Input: part model. Units: mm. Frame: model coordinates. A direction names the side the tool comes from. Coordinates: 2 decimals unless noted, no trailing zeros. Put each result on its own line as item: value. Start each with the question number.
1) Contact query for flat-ended pins moving along their axis: P1, Ø2, axis at x = -1.5, y = -1, coming from the -Z side; P2, Ø3, axis at x = 4, y = -3, coming from the +Z side; P3, Ø2, axis at y = 1.5, z = 10, coming from the +X side; P4, Ø1, axis at y = -7, z = 12, coming from the -X side. Output: stop coordinate, or through.
2) Material intervals for L1, parallel to Y at x = -3, z = 9.5; L2, parallel to Y at x = 3.25, z = 1.5; L3, parallel to X at y = -2.25, z = 4.25, sorted ascending.
3) Set-up query: faces 4 (the flat face through (-4, 0, 5)), 5 (the cylindrical face through (-1.859, -9.919, 24.032)), 6 (the cylindrical face through (3.098, -6.416, 20.157)), 7 (the cylindrical face through (-1.941, -3.786, 27.573)), 8 (the cylindrical face through (4.241, -6.849, 25.805)). Return all of +Z, -Z, +X, -X, +Y, -Y with unobstructed straight access to the full face (end or side cutting, diameter ignored); none if empty.
4) Pull-direction query (X, two-part tool) for faces 1 (the cylindrical face through (3.1, 2.44, 5.34)), 2 (the flat face through (-5.05, -6.98, 25.99)), 3 (the cylindrical face through (5.359, -6.849, 25.805)); classes: pulls with the +X half, pulls with the -X half, needs draft (parallel to the pull), parting line crosses it, or undercut.
from build123d import *

# Parameters (mm, degrees)
CUT_EXTRUDE1_DEPTH = 10
CUT_EXTRUDE2_DEPTH = 10
FILLET1_R          = 0.8


with BuildPart() as part:
    # Sweep1: sweep along a path in Sketch2
    with BuildLine(Plane(origin=(0, 0, 0), x_dir=(0, 0, -1), z_dir=(1, 0, 0))) as sweep1_path:
        Line((0, 0), (-10, 0))
        ThreePointArc((-10, 0), (-13.799332082, -0.500191558), (-17.339745962, -1.966679003))
        Line((-17.339745962, -1.966679003), (-26, -6.966679003))
    # Sketch1 → Sweep1 (sweep)
    with BuildSketch(Plane.XY):
        with BuildLine():
            Line((-5.6, 4.9), (1, 4.9))
            ThreePointArc((1, 4.9), (4.252691193, 3.552691193), (5.6, 0.3))
            Line((5.6, 0.3), (5.6, -0.3))
            ThreePointArc((5.6, -0.3), (4.252691193, -3.552691193), (1, -4.9))
            Line((1, -4.9), (-5.6, -4.9))
            Line((-5.6, -4.9), (-5.6, 4.9))
        make_face()
        Polygon((2.655811238, 0), (1.327905619, 2.3), (-1.327905619, 2.3), (-2.655811238, 0), (-1.327905619, -2.3), (1.327905619, -2.3), align=None, mode=Mode.SUBTRACT)
    sweep(path=sweep1_path.line)

    # Sketch3 → Cut-Extrude1 (cut)
    with BuildSketch(Plane(origin=(0, 0, 0), x_dir=(-1, 0, 0), z_dir=(0, 0, -1))):
        with BuildLine():
            Line((4, -3.3), (4, 3.3))
            Line((4, 3.3), (-1, 3.3))
            ThreePointArc((-1, 3.3), (-3.121320344, 2.421320344), (-4, 0.3))
            Line((-4, 0.3), (-4, -0.3))
            ThreePointArc((-4, -0.3), (-3.121320344, -2.421320344), (-1, -3.3))
            Line((-1, -3.3), (4, -3.3))
        make_face()
    extrude(amount=-CUT_EXTRUDE1_DEPTH, mode=Mode.SUBTRACT)

    # Sketch4 → Cut-Extrude2 (cut)
    with BuildSketch(Plane(origin=(0, -13, 22.516660498), x_dir=(1, 0, 0), z_dir=(0, -0.5000000000000009, 0.8660254037844382))):
        with BuildLine():
            Line((-4, 10.266679003), (-4, 3.666679003))
            Line((-4, 3.666679003), (1, 3.666679003))
            ThreePointArc((1, 3.666679003), (3.121320344, 4.54535866), (4, 6.666679003))
            Line((4, 6.666679003), (4, 7.266679003))
            ThreePointArc((4, 7.266679003), (3.121320344, 9.387999347), (1, 10.266679003))
            Line((1, 10.266679003), (-4, 10.266679003))
        make_face()
    extrude(amount=-CUT_EXTRUDE2_DEPTH, mode=Mode.SUBTRACT)

    # Fillet1
    fillet1_edges = [part.edges().sort_by_distance(p)[0] for p in [
        (-1.5, -4.108795171, 27.65),
        (-4, -6.966679003, 26),
        (-1.5, -9.824562836, 24.35),
        (3.121320344, -9.063603931, 24.789339828),
        (4, -6.966679003, 26),
        (3.121320344, -4.869754075, 27.210660172),
        (-2.3, 4.9, 0),
        (4.252691193, 3.552691193, 0),
        (5.6, 0, 0),
        (4.252691193, -3.552691193, 0),
        (-2.3, -4.9, 0),
        (-2.3, -2.723154525, 28.45),
        (4.252691193, -3.889958178, 27.776345597),
        (5.6, -6.966679003, 26),
        (4.252691193, -10.043399829, 24.223654403),
        (-2.3, -11.210203482, 23.55),
        (-1.5, -3.3, 0),
        (-4, 0, 0),
        (-1.5, 3.3, 0),
        (3.121320344, 2.421320344, 0),
        (4, 0, 0),
        (3.121320344, -2.421320344, 0),
    ]]
    fillet(fillet1_edges, radius=FILLET1_R - 0.0001)  # a hair under: the kernel refuses the full size


solid = part.part
Results found:
1. P1: stops at z = 10
1. P2: stops at z = 28.02
1. P3: stops at x = 5.6
1. P4: passes through
2. L1: y = -4.9 to -3.3, 3.3 to 4.9
2. L2: y = -4.31 to -2.28, 2.28 to 4.31
2. L3: x = -5.6 to -4, 3.28 to 5.17
3. face 4: -Z
3. face 5: +Z
3. face 6: none
3. face 7: -Y
3. face 8: +Z, -Y
4. face 1: undercut
4. face 2: needs draft
4. face 3: pulls with the +X half
